```python
from build123d import *
from OCP.BRepFilletAPI import BRepFilletAPI_MakeChamfer

# Parameters (mm, degrees)
SKETCH1_R               = 14.5
BOSS_EXTRUDE1_DEPTH     = 7
BOSS_EXTRUDE2_DEPTH     = 2
BOSS_EXTRUDE3_DEPTH     = 5
CHAMFER1_SIZE           = 5
CHAMFER1_SIZE2          = 3.942733198
CUT_EXTRUDE1_REACH      = 134.354
CUT_EXTRUDE1_END_RADIUS = 14.5
CUT_EXTRUDE1_START      = -1
SKETCH3_W               = 6.1
SKETCH3_H               = 6.1
SKETCH3_R               = 2.35
SKETCH3_3_R             = 2.35
CUT_EXTRUDE2_DEPTH      = 5


with BuildPart() as part:
    # Sketch1 → Boss-Extrude1 (new body)
    with BuildSketch(Plane(origin=(0, 0, 0), x_dir=(-1, 0, 0), z_dir=(0, 0, -1))):
        Polygon((-132.76, -106.571268837), (-132.76, -84.748729163), (-144.048730163, -73.459999), (-165.871269837, -73.459999), (-177.16, -84.748729163), (-177.16, -106.571268837), (-165.871269837, -117.859999), (-144.048730163, -117.859999), align=None)
        with Locations((-154.96, -95.659999)):
            Circle(SKETCH1_R, mode=Mode.SUBTRACT)
    extrude(amount=BOSS_EXTRUDE1_DEPTH)

    # Sketch1<3> → Boss-Extrude2 (add)
    with BuildSketch(Plane(origin=(0, 0, 0), x_dir=(-1, 0, 0), z_dir=(0, 0, -1))):
        Polygon((-165.871269837, -117.859999), (-144.048730163, -117.859999), (-132.76, -106.571268837), (-132.76, -84.748729163), (-144.048730163, -73.459999), (-165.871269837, -73.459999), (-177.16, -84.748729163), (-177.16, -106.571268837), align=None)
        Polygon((-134.76, -85.577156288), (-144.877157288, -75.459999), (-165.042842712, -75.459999), (-175.16, -85.577156288), (-175.16, -105.742841712), (-165.042842712, -115.859999), (-144.877157288, -115.859999), (-134.76, -105.742841712), align=None, mode=Mode.SUBTRACT)
    extrude(amount=-BOSS_EXTRUDE2_DEPTH)

    # Sketch2 → Boss-Extrude3 (add)
    with BuildSketch(Plane.XY.offset(-7)):
        Polygon((142.46, -70.659999), (167.46, -70.659999), (168.84199674, -73.459999), (171.737289726, -79.326018889), (177.16, -84.748729163), (168.84199674, -67.896005521), (141.07800326, -67.896005521), (132.76, -84.748729163), (138.182710274, -79.326018889), (141.07800326, -73.459999), align=None)
    boss_extrude3 = extrude(amount=BOSS_EXTRUDE3_DEPTH)

    # Chamfer1: one chamfer whose edges measure the first distance from different faces: ONE call of the kernel's chamfer builder (chamfer() names one face for all edges)
    chamfer1_edges_1 = [part.edges().sort_by_distance(p)[0] for p in [
        (171.737289726, -79.326018889, -4.5),
    ]]
    chamfer1_side_1 = [part.faces().sort_by_distance(p)[0] for p in [
        (169.598644863, -74.993008944, -4.5),
    ]]
    chamfer1_edges_2 = [part.edges().sort_by_distance(p)[0] for p in [
        (138.182710274, -79.326018889, -4.5),
    ]]
    chamfer1_side_2 = [part.faces().sort_by_distance(p)[0] for p in [
        (139.472020238, -78.036708925, -1.77197304),
    ]]
    chamfer1 = BRepFilletAPI_MakeChamfer(part.part.solid().wrapped)
    for e in chamfer1_edges_1:
        chamfer1.Add(CHAMFER1_SIZE, CHAMFER1_SIZE2, e.wrapped, chamfer1_side_1[0].wrapped)  # the first distance lies on this face
    for e in chamfer1_edges_2:
        chamfer1.Add(CHAMFER1_SIZE, CHAMFER1_SIZE2, e.wrapped, chamfer1_side_2[0].wrapped)  # the first distance lies on this face
    add(Compound.cast(chamfer1.Shape()), mode=Mode.REPLACE)

    # Mirror1: Boss-Extrude3 across plane
    add(boss_extrude3.mirror(Plane(origin=(0, -95.659999, 0), x_dir=(0, 0, 1), z_dir=(0, -1, 0))))

    # Cut-Extrude1: up to this cylinder (the profile starts outside it)
    cut_extrude1_end = Plane(origin=(154.96, -95.659999, -1.5681335), z_dir=(0, 0, 1)) * Cylinder(CUT_EXTRUDE1_END_RADIUS, 301.671733, mode=Mode.PRIVATE)
    # Sketch3 → Cut-Extrude1 (cut, up to the surface)
    with BuildSketch(Plane.ZY.offset(-132.76).offset(CUT_EXTRUDE1_START), mode=Mode.PRIVATE) as cut_extrude1_sk1:
        with Locations((-3.05, -95.659999)):
            Rectangle(SKETCH3_W, SKETCH3_H)
        with Locations((-3.05, -95.659999)):
            Circle(SKETCH3_R, mode=Mode.SUBTRACT)
    cut_extrude1_tool1 = extrude(cut_extrude1_sk1.sketch, amount=-CUT_EXTRUDE1_REACH, mode=Mode.PRIVATE) - cut_extrude1_end
    add(cut_extrude1_tool1.solids().sort_by_distance((133.76, -95.659999, -0.086267))[0], mode=Mode.SUBTRACT)
    # Sketch3 → Cut-Extrude1 (cut, up to the surface)
    with BuildSketch(Plane.ZY.offset(-132.76).offset(CUT_EXTRUDE1_START), mode=Mode.PRIVATE) as cut_extrude1_sk2:
        with Locations((-3.05, -95.659999)):
            Circle(SKETCH3_R)
    cut_extrude1_tool2 = extrude(cut_extrude1_sk2.sketch, amount=-CUT_EXTRUDE1_REACH, mode=Mode.PRIVATE) - cut_extrude1_end
    add(cut_extrude1_tool2.solids().sort_by_distance((133.76, -95.659999, -3.05))[0], mode=Mode.SUBTRACT)

    # Sketch3<3> → Cut-Extrude2 (cut)
    with BuildSketch(Plane.ZY.offset(-132.76)):
        with Locations((-3.05, -95.659999)):
            Circle(SKETCH3_3_R)
    extrude(amount=-CUT_EXTRUDE2_DEPTH, mode=Mode.SUBTRACT)


solid = part.part
```
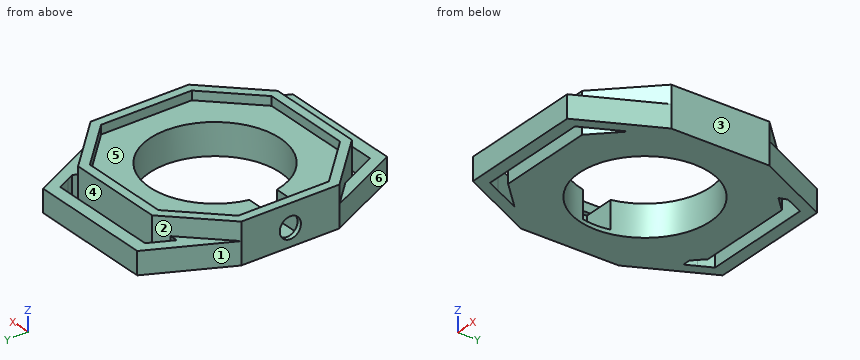
The listing builds one solid part. Answer for the finished solid, in the listing's coordinates (mm). Face numbers are marked on the shaded views. A direction names the side the tool comes from. Coordinates: 2 decimals unless noted, no trailing zeros. Write each loop counter-clockwise with the first axis right and the second up, starting at its lowest first coordinate (ties: lowest second). Pieces come first, ordered by that corner, then holes.
Q1. The mould has two halves that part along Y. Classify the marked faces 1, 2 and 3: released by +Y, released by -Y, zero draft, split by the parting line, or undercut.
Returned:
face 1: released by +Y
face 2: undercut
face 3: zero draft
Q2. Section D-D, the plane y = -114 is taken. Write down the section's boundary in (x, z), then the cut area to 3 significant figures.
Returned:
outline: (136.43, -7) - (139.17, -7) - (139.17, -2) - (136.43, -2) - close; (140.19, -7) - (169.73, -7) - (169.73, 2) - (166.9, 2) - (166.9, 0) - (143.02, 0) - (143.02, 2) - (140.19, 2) - close; (170.75, -7) - (173.49, -7) - (173.49, -2) - (170.75, -2) - close
area: 246 mm2
Q3. Section B-B, the plane y = -103.5 is taken. Write down the section's boundary in (x, z), then the cut area to 3 significant figures.
Returned:
outline: (132.76, -7) - (142.76, -7) - (142.76, 0) - (134.76, 0) - (134.76, 2) - (132.76, 2) - close; (167.16, -7) - (177.16, -7) - (177.16, 2) - (175.16, 2) - (175.16, 0) - (167.16, 0) - close
area: 148 mm2
Q4. Section A-A, the plane x = 154.96 is taken. Write down the section's boundary in (y, z), then the cut area to 3 significant figures.
Returned:
outline: (-123.42, -7) - (-120.66, -7) - (-120.66, -2) - (-123.42, -2) - close; (-117.86, -7) - (-110.16, -7) - (-110.16, 0) - (-115.86, 0) - (-115.86, 2) - (-117.86, 2) - close; (-81.16, -7) - (-73.46, -7) - (-73.46, 2) - (-75.46, 2) - (-75.46, 0) - (-81.16, 0) - close; (-70.66, -7) - (-67.9, -7) - (-67.9, -2) - (-70.66, -2) - close
area: 143 mm2
Q5. Which of the six approach directions +Z, -Z, +X, -X, +Y, -Y give full straight-line access (tool end or side, diameter ignored) to the marked faces 4, 5 and 6?
Returned:
face 4: +Z, -Z
face 5: +Z
face 6: +Z, -Z, -X, -Y
Q6. Given P1, Ø1, axis at x = 151.5, z = 0.5, coming from the +Y side; P2, Ø5, axis at x = 137.5, y = -97, coming from the +Z side; P3, Ø5, axis at x = 170, z = -3, coming from the -Y side; P4, Ø4, axis at x = 138, z = -1, coming from the +Y side, each flat-ended and moving along its own axis, determine where each tip first touches the part or whether it passes through.
Returned:
P1: stops at y = -73.46
P2: stops at z = 0
P3: stops at y = -123.42
P4: stops at y = -70.62
Q7. Find the intervals of material crossed by line 1 along Y through (x, z) = (158, -6); line 2 along Y through (x, z) = (152.5, 1.5); line 3 along X through (y, z) = (-112.5, -6.5), in increasing order.
Returned:
line 1: y = -123.42 to -120.66, -117.86 to -109.84, -81.48 to -73.46, -70.66 to -67.9
line 2: y = -117.86 to -115.86, -75.46 to -73.46
line 3: x = 135.69 to 138.43, 138.69 to 171.23, 171.49 to 174.23
Q8. Section C-C, the plane z = -3 is taken. Give the number of separate pieces and of enclosed holes in the cut face, then the cut area to 3 significant figures.
Returned:
separate pieces: 1
enclosed holes: 2
area: 1,300 mm2
